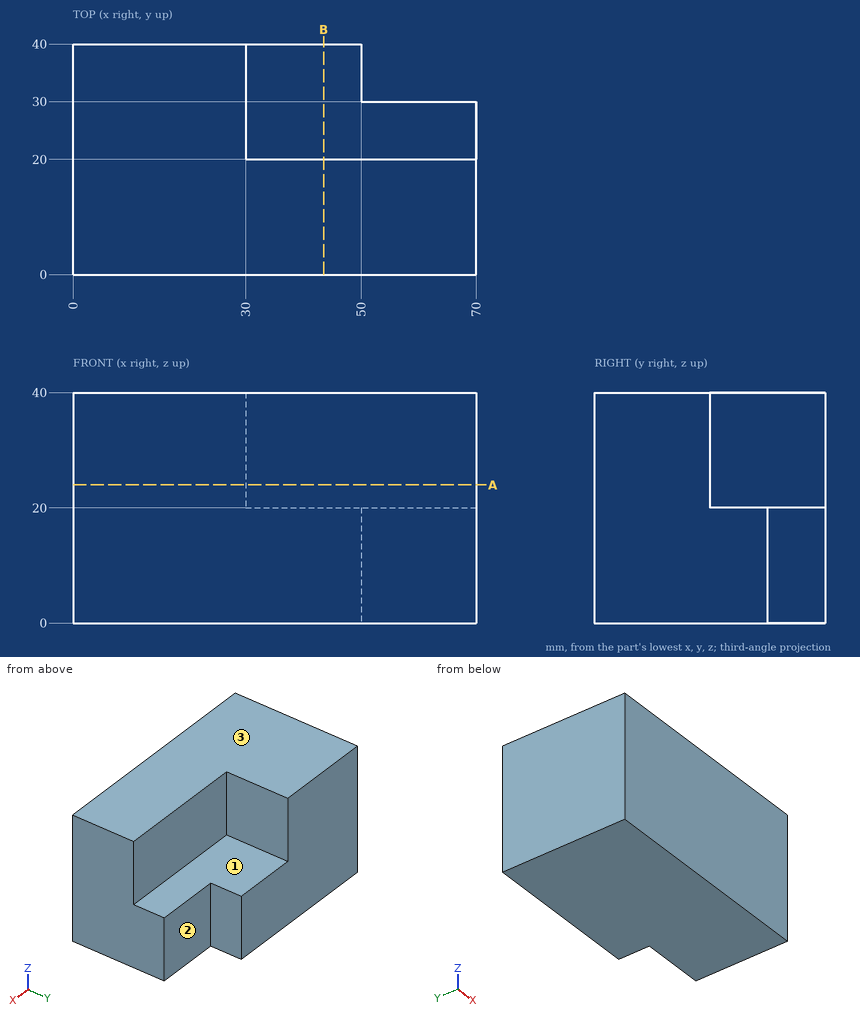
Input: dimensioned drawing with shaded views. Units: mm. Origin: part minimum x, y, z. A direction names the side the tool comes from. Give positions to 0.01 mm unless a question says otherwise; leave off trailing zeros. Write each loop counter-clockwise with the first axis right and the second up, starting at its lowest first coordinate (ties: lowest second). Pieces come first, ordered by that corner, then holes.
1. Line query: probe 1 along Y at (x, z) = (47.5, 21.5); probe 2 along X at (y, z) = (21, 27). Output: solid intervals per line, ascending.
2. Section query A-A, the plane z = 24. Return loops of the section in (x, y), then the cut area to 3 significant figures.
3. Section query B-B, the plane x = 43.5. Return loops of the section in (y, z), then the cut area to 3 significant figures.
4. Pin query (flat end, axial travel): P1, Ø16, axis at x = 55.5, z = 10.5, coming from the +Y side; P2, Ø10, axis at y = 25.5, z = 28.5, coming from the +X side; P3, Ø8, axis at y = 37.5, z = 8.5, coming from the +X side; P4, Ø22, axis at x = 44, z = 33.5, coming from the +Y side. Return the tip coordinate at first contact, or that it passes through.
5. Reachability of the marked faces 1, 2 and 3 from +Z, -Z, +X, -X, +Y, -Y: full face, straight path, thin tool, end or side. Return the list, or none.
Computed:
1. probe 1: y = 0 to 20
1. probe 2: x = 0 to 30
2. outline: (0, 0) - (70, 0) - (70, 20) - (30, 20) - (30, 40) - (0, 40) - close
2. area: 2,000 mm2
3. outline: (0, 0) - (40, 0) - (40, 20) - (20, 20) - (20, 40) - (0, 40) - close
3. area: 1,200 mm2
4. P1: stops at y = 40
4. P2: stops at x = 30
4. P3: stops at x = 50
4. P4: stops at y = 20
5. face 1: +Z, +X, +Y
5. face 2: +Z, -Z, +X, +Y
5. face 3: +Z, +X, -X, +Y, -Y
